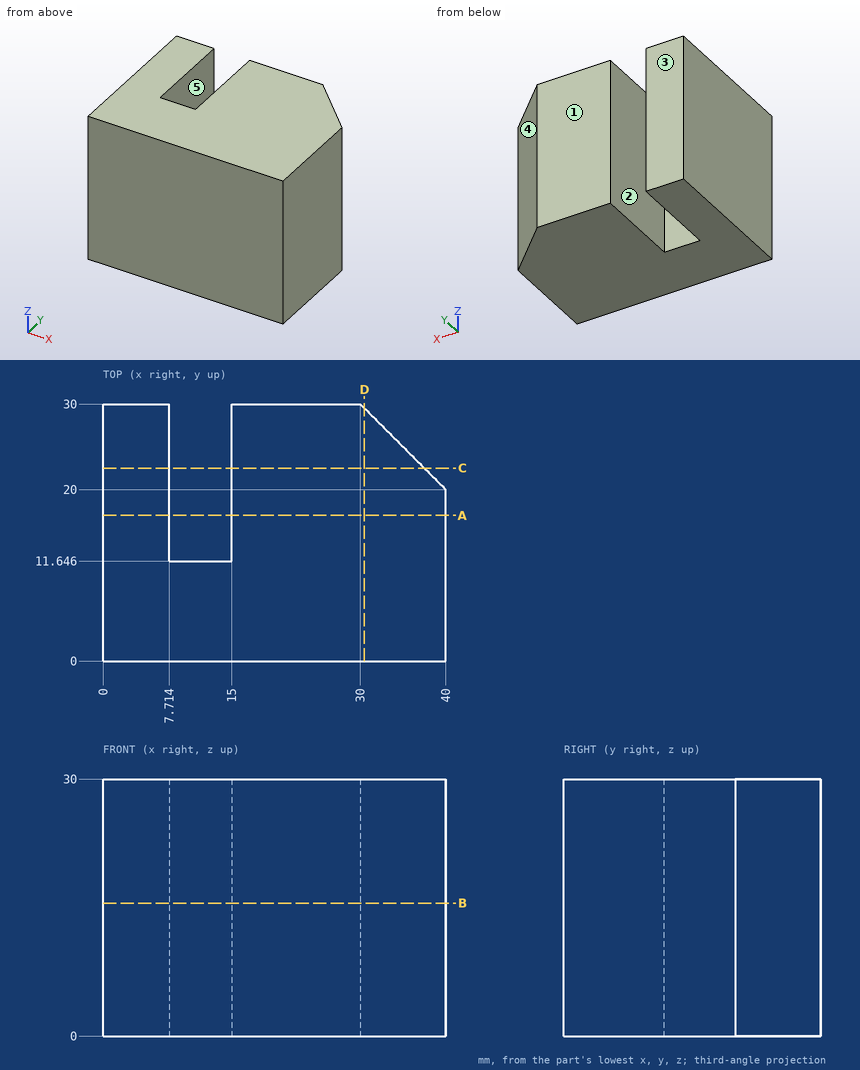
Can you work these out from the drawing? Everything is in mm from the part's minimum corner. A direction names the side the tool comes from. Give positions to 0.01 mm unless a question says otherwise; leave off trailing zeros. Order: outer loops, then holes, each group sorted by start corner. A loop starts at its lowest first (then second) coordinate and runs counter-clockwise, first axis right, second up. Notation, with made-up numbers: M 72.5,36.25 L 117.5,36.25 A19 cw 117.5,51.25 Z; hole C 36.5,-38.75 d6. An arc over 180 degrees is marked long. Write item = value, one per line. Start each with the question number.
Q1. Suppose I cut it at D-D (x = 30.5). Write out the boundary of the cut face in (y, z), plus the area to 3 significant figures.
Q2. We'd pull the mould along X, two halves only. Please class the marked faces 3, 4 and 5: pulls with the +X half, pulls with the -X half, needs draft (parallel to the pull), parting line crosses it, or undercut.
Q3. Suppose I cut it at C-C (y = 22.5). Write out the boundary of the cut face in (x, z) (1 decimal).
Q4. For the marked faces 1 and 2, which set-ups out of +Z, -Z, +X, -X, +Y, -Y let a thin tool reach every point of the face, with its end or its side?
Q5. Will these pins go through, and if not, where does the flat tip stop? pin 1 Ø2 at (x, z) = (12.5, 9.5) entering from +Y; pin 2 Ø4 at (y, z) = (22.5, 22) entering from +X.
Q6. Suppose I cut it at B-B (z = 15.5). Write out the boundary of the cut face in (x, y) (1 decimal).
Q7. I need wall thicknesses on probe 1 along X at (y, z) = (18.75, 22) (1 decimal); probe 2 along Y at (x, z) = (13.5, 10); probe 3 along X at (y, z) = (28.5, 11) (1 decimal). Which ranges of each line are inside material? Lowest first, please. Write a range as [from, to].
Q8. Suppose I cut it at A-A (y = 17). Write out the boundary of the cut face in (x, z) (1 decimal).
Check result:
q1.outline = M 0,0 L 29.5,0 L 29.5,30 L 0,30 Z
q1.area = 885 mm2
q2.face_3 = needs draft
q2.face_4 = pulls with the +X half
q2.face_5 = undercut
q3.outline = M 0,0 L 7.7,0 L 7.7,30 L 0,30 Z; M 15,0 L 37.5,0 L 37.5,30 L 15,30 Z
q4.face_1 = +Z, -Z, +X, -X, +Y
q4.face_2 = +Z, -Z, +Y
q5.pin_1 = 11.65
q5.pin_2 = 39.5
q6.outline = M 0,0 L 40,0 L 40,20 L 30,30 L 15,30 L 15,11.6 L 7.7,11.6 L 7.7,30 L 0,30 Z
q7.probe_1 = [0, 7.7], [15, 40]
q7.probe_2 = [0, 11.65]
q7.probe_3 = [0, 7.7], [15, 31.5]
q8.outline = M 0,0 L 7.7,0 L 7.7,30 L 0,30 Z; M 15,0 L 40,0 L 40,30 L 15,30 Z
